Read the model definition and answer for the solid it produces. Units are mm, in the model's axes. Give positions to 0.01 mm unless a question says otherwise; leave off trailing zeros. Loops run counter-clockwise (first coordinate to the right, second up) from the corner with the lowest first, then second, coordinate; pieces in that order, holes last. Notation, with made-up numbers: (51.5, 52.5) -> (89.5, 52.5) arc R16 ccw to (89.5, 65.5) -> close; hole circle Ø10 at (20.25, 59.5). An arc over 180 degrees is marked (long way). Write each question's results on one line, items separated by ' | '. Start each with the question number.
Item 1: Section C-C on x = 0.65 is taken. State how many separate pieces and enclosed holes the cut face has, and give its area (3 significant figures).
Item 2: Section B-B on z = 21 is taken. Write down the section's boundary in (x, y).
Item 3: Section A-A on y = 51.6 is taken. Write down the section's boundary in (x, z).
Item 4: Section D-D on y = -27 is taken. Write down the section's boundary in (x, z).
Item 5: Find the intervals of material crossed by line 1 (Z direction, x = 1.55, y = 44); line 2 (Y direction, x = 0.95, z = -32); line 3 (Z direction, x = 1.45, y = -17), in increasing order.
Item 6: Each of these flat-tipped pins is pushed along its axis until it touches: P1, Ø1, axis at x = 1, y = -10, coming from the +Z side; P2, Ø7.5, axis at y = 41.75, z = -30.33, coming from the +X side. Where does it stop, or does it pass through?
```python
from build123d import *

# Parameters (mm, degrees)
SKETCH3_R          = 0.25
CUT_EXTRUDE1_DEPTH = 85.876380696
SKETCH4_R          = 3.25
CUT_EXTRUDE2_DEPTH = 10


with BuildPart() as part:
    # Sketch2 → Revolve1 (revolve)
    with BuildSketch(Plane.XY, mode=Mode.PRIVATE) as revolve1_sk:
        Polygon((2, 0), (2, 31), (2, 60), (0, 60), (0, 0), align=None)
    revolve(revolve1_sk.sketch.rotate(Axis((0, 0, 0), (1, 0, 0)), 90), axis=Axis((0, 0, 0), (1, 0, 0)))

    # Sketch3 → Cut-Extrude1 (cut, through all)
    with BuildSketch(Plane.ZY):
        Circle(SKETCH3_R)
        with Locations((0, 9)):
            Circle(SKETCH3_R)
        with Locations((0, 17)):
            Circle(SKETCH3_R)
        with Locations((0, 25)):
            Circle(SKETCH3_R)
        with Locations((7.794228634, 4.5)):
            Circle(SKETCH3_R)
        with Locations((7.794228634, -4.5)):
            Circle(SKETCH3_R)
        with Locations((0, -9)):
            Circle(SKETCH3_R)
        with Locations((-7.794228634, -4.5)):
            Circle(SKETCH3_R)
        with Locations((-7.794228634, 4.5)):
            Circle(SKETCH3_R)
        with Locations((8.5, 14.722431864)):
            Circle(SKETCH3_R)
        with Locations((14.722431864, 8.5)):
            Circle(SKETCH3_R)
        with Locations((17, 0)):
            Circle(SKETCH3_R)
        with Locations((14.722431864, -8.5)):
            Circle(SKETCH3_R)
        with Locations((8.5, -14.722431864)):
            Circle(SKETCH3_R)
        with Locations((0, -17)):
            Circle(SKETCH3_R)
        with Locations((-8.5, -14.722431864)):
            Circle(SKETCH3_R)
        with Locations((-14.722431864, -8.5)):
            Circle(SKETCH3_R)
        with Locations((-17, 0)):
            Circle(SKETCH3_R)
        with Locations((-14.722431864, 8.5)):
            Circle(SKETCH3_R)
        with Locations((-8.5, 14.722431864)):
            Circle(SKETCH3_R)
        with Locations((9.567085809, 23.096988313)):
            Circle(SKETCH3_R)
        with Locations((17.67766953, 17.67766953)):
            Circle(SKETCH3_R)
        with Locations((23.096988313, 9.567085809)):
            Circle(SKETCH3_R)
        with Locations((25, 0)):
            Circle(SKETCH3_R)
        with Locations((23.096988313, -9.567085809)):
            Circle(SKETCH3_R)
        with Locations((17.67766953, -17.67766953)):
            Circle(SKETCH3_R)
        with Locations((9.567085809, -23.096988313)):
            Circle(SKETCH3_R)
        with Locations((0, -25)):
            Circle(SKETCH3_R)
        with Locations((-9.567085809, -23.096988313)):
            Circle(SKETCH3_R)
        with Locations((-17.67766953, -17.67766953)):
            Circle(SKETCH3_R)
        with Locations((-23.096988313, -9.567085809)):
            Circle(SKETCH3_R)
        with Locations((-25, 0)):
            Circle(SKETCH3_R)
        with Locations((-23.096988313, 9.567085809)):
            Circle(SKETCH3_R)
        with Locations((-17.67766953, 17.67766953)):
            Circle(SKETCH3_R)
        with Locations((-9.567085809, 23.096988313)):
            Circle(SKETCH3_R)
    extrude(amount=-CUT_EXTRUDE1_DEPTH, mode=Mode.SUBTRACT)

    # Sketch4 → Cut-Extrude2 (cut)
    with BuildSketch(Plane.ZY):
        with Locations((0, 51.6)):
            Circle(SKETCH4_R)
        with Locations((30.329719018, 41.74527691)):
            Circle(SKETCH4_R)
        with Locations((49.074516241, 15.94527691)):
            Circle(SKETCH4_R)
        with Locations((49.074516241, -15.94527691)):
            Circle(SKETCH4_R)
        with Locations((30.329719018, -41.74527691)):
            Circle(SKETCH4_R)
        with Locations((0, -51.6)):
            Circle(SKETCH4_R)
        with Locations((-30.329719018, -41.74527691)):
            Circle(SKETCH4_R)
        with Locations((-49.074516241, -15.94527691)):
            Circle(SKETCH4_R)
        with Locations((-49.074516241, 15.94527691)):
            Circle(SKETCH4_R)
        with Locations((-30.329719018, 41.74527691)):
            Circle(SKETCH4_R)
    extrude(amount=-CUT_EXTRUDE2_DEPTH, mode=Mode.SUBTRACT)


solid = part.part
```
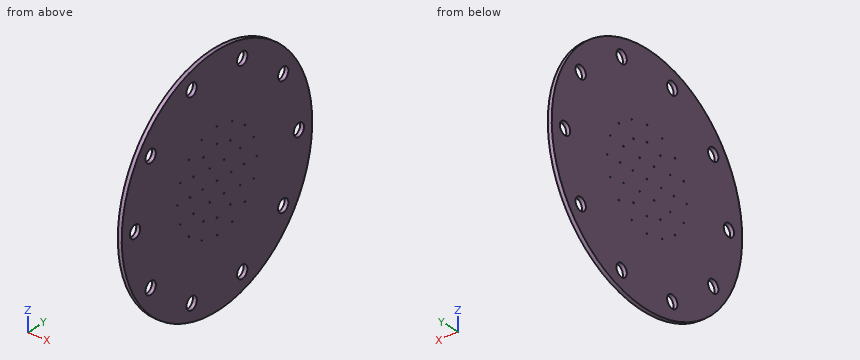
Findings:
1) separate pieces: 1 | enclosed holes: 45 | area: 11,000 mm2
2) outline: (0, -56.2) -> (2, -56.2) -> (2, 56.2) -> (0, 56.2) -> close
3) outline: (0, -30.62) -> (2, -30.62) -> (2, -3.25) -> (0, -3.25) -> close; (0, 3.25) -> (2, 3.25) -> (2, 30.62) -> (0, 30.62) -> close
4) outline: (0, -53.58) -> (2, -53.58) -> (2, 53.58) -> (0, 53.58) -> close
5) line 1: -40.79 to -32.67, -27.99 to 27.99, 32.67 to 40.79 | line 2: -50.75 to -44.53, -38.96 to 38.96, 44.53 to 50.75 | line 3: -57.54 to -52.15, -46 to -0.25, 0.25 to 46, 52.15 to 57.54
6) P1: z = 59.24 | P2: x = 2
